Here's how the part is built. I have some questions about the finished solid (model axes, mm). Give positions to 0.01 mm unless a question says otherwise; leave off trailing zeros. Loops run counter-clockwise (first coordinate to the right, second up) from the corner with the lowest first, then second, coordinate; pieces in that order, holes last.
Q1. I need wall thicknesses on probe 1 along Z at (x, y) = (20.5, 3); probe 2 along Z at (x, y) = (0, 4.75); probe 3 along Z at (x, y) = (88, 1). Which ranges of each line are inside material? Lowest first, please.
Q2. I'm going to push flat-ended pins straight in: P1, Ø1, axis at y = 2, z = -40, coming from the +X side; P2, Ø2, axis at y = 3, z = -9, coming from the +X side; P3, Ø3, axis at x = 110, y = 2, coming from the +Z side; P4, Ø4, axis at x = 17.64, z = -49.39, coming from the +Y side. Where does each tip first touch, or does it pass through?
Q3. Suppose I cut it at B-B (z = 0). List the corners of the cut face in (x, y) for me, and give its area (3 significant figures).
Q4. Suppose I cut it at A-A (x = 79.5). List the corners of the cut face in (y, z) for me, and give its area (3 significant figures).
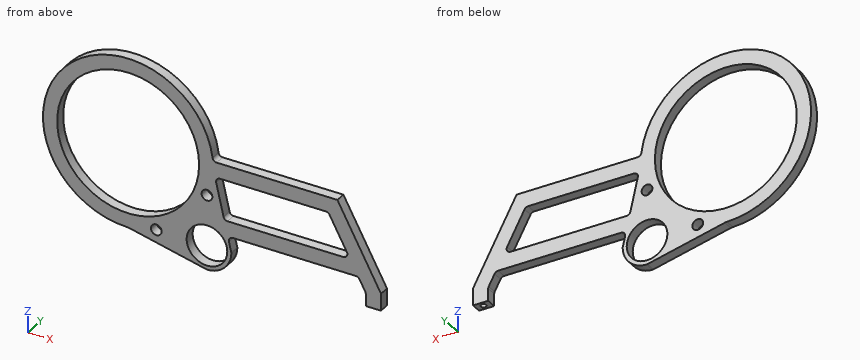
```python
from build123d import *

# Parameters (mm, degrees)
BOSS_EXTRUDE1_DEPTH             = 6.35
FILLET2_R                       = 6.35
BOSS_EXTRUDE2_DEPTH             = 6.35
SKETCH3_R                       = 44.4754
SKETCH3_R_2                     = 12.7254
CUT_EXTRUDE1_DEPTH              = 7.35
FILLET3_R                       = 2.54
F_6_32_TAPPED_HOLE1_D           = 2.7051
F_6_32_TAPPED_HOLE1_DEPTH       = 9.398
F_6_32_TAPPED_HOLE1_CBORE_D     = 3.5052
F_6_32_TAPPED_HOLE1_CBORE_DEPTH = 7.112
F_6_32_TAPPED_HOLE1_TIP         = 0.81269403
F_1_4_CLEARANCE_HOLE1_D         = 6.7564
F_1_4_CLEARANCE_HOLE1_DEPTH     = 25.4
F_1_4_CLEARANCE_HOLE1_TIP       = 2.029827343


with BuildPart() as part:
    # Sketch1 → Boss-Extrude1 (new body)
    with BuildSketch(Plane(origin=(0, 0, 0), x_dir=(1, 0, 0), z_dir=(0, 1, 0))):
        with BuildLine():
            Line((0, 53.3781), (49.391408666, 64.669508666))
            ThreePointArc((49.391408666, 64.669508666), (60.19465678, 60.19465678), (64.669508666, 49.391408666))
            Line((64.669508666, 49.391408666), (53.3781, 0))
            ThreePointArc((53.3781, 0), (-37.744016477, -37.744016477), (0, 53.3781))
        make_face()
    extrude(amount=BOSS_EXTRUDE1_DEPTH)

    # Fillet2
    fillet2_edges = [part.edges().sort_by_distance(p)[0] for p in [
        (0, 3.175, -53.3781),
        (53.3781, 3.175, 0),
    ]]
    fillet(fillet2_edges, radius=FILLET2_R)

    # Sketch4 → Boss-Extrude2 (add)
    with BuildSketch(Plane(origin=(0, 6.35, 0), x_dir=(1, 0, 0), z_dir=(0, 1, 0))):
        Polygon((52.07, -4.84480564), (131.116478857, -4.84480564), (158.4325, 45.95519436), (158.4325, 56.6794421), (148.9075, 56.6794421), (148.9075, 48.353689839), (144.203285679, 39.60519436), (52.07, 39.60519436), (52.07, 30.08019436), (139.081531715, 30.08019436), (125.423521143, 4.68019436), (52.07, 4.68019436), align=None)
    extrude(amount=-BOSS_EXTRUDE2_DEPTH)

    # Sketch3 → Cut-Extrude1 (cut, through all)
    with BuildSketch(Plane(origin=(0, 6.35, 0), x_dir=(1, 0, 0), z_dir=(0, 1, 0))):
        Circle(SKETCH3_R)
        with Locations((49.391408666, 49.391408666)):
            Circle(SKETCH3_R_2)
    extrude(amount=-CUT_EXTRUDE1_DEPTH, mode=Mode.SUBTRACT)

    # Fillet3
    fillet3_edges = [part.edges().sort_by_distance(p)[0] for p in [
        (139.081531715, 3.175, -30.08019436),
        (54.448042903, 3.175, -4.68019436),
        (125.423521143, 3.175, -4.68019436),
        (60.25475682, 3.175, -30.08019436),
        (62.432274539, 3.175, -39.60519436),
        (144.203285679, 3.175, -39.60519436),
        (148.9075, 3.175, -48.353689839),
        (53.157778527, 3.175, 4.84480564),
        (49.391408666, 3.175, -64.669508666),
        (64.669508666, 3.175, -49.391408666),
    ]]
    fillet(fillet3_edges, radius=FILLET3_R)

    # #6-32 Tapped Hole1
    with Locations(Plane(origin=(0, 0, -56.6794421), x_dir=(-1, 0, 0), z_dir=(0, 0, -1))):
        with Locations((-153.67, 3.175)):
            CounterBoreHole(F_6_32_TAPPED_HOLE1_D / 2, F_6_32_TAPPED_HOLE1_CBORE_D / 2, F_6_32_TAPPED_HOLE1_CBORE_DEPTH, depth=F_6_32_TAPPED_HOLE1_DEPTH)
            with Locations((0, 0, -(F_6_32_TAPPED_HOLE1_DEPTH + F_6_32_TAPPED_HOLE1_TIP / 2))):  # 118° drill point
                Cone(0, F_6_32_TAPPED_HOLE1_D / 2, F_6_32_TAPPED_HOLE1_TIP, mode=Mode.SUBTRACT)

    # 1/4 Clearance Hole1
    with Locations(Plane.XZ):
        with Locations((49.391408666, -17.641408666), (17.641408666, -49.391408666)):
            Hole(F_1_4_CLEARANCE_HOLE1_D / 2, depth=F_1_4_CLEARANCE_HOLE1_DEPTH)
            with Locations((0, 0, -(F_1_4_CLEARANCE_HOLE1_DEPTH + F_1_4_CLEARANCE_HOLE1_TIP / 2))):  # 118° drill point
                Cone(0, F_1_4_CLEARANCE_HOLE1_D / 2, F_1_4_CLEARANCE_HOLE1_TIP, mode=Mode.SUBTRACT)


solid = part.part
```
Solutions:
1. probe 1: z = -58.06 to -51.19, -47.59 to -39.47, 39.47 to 49.28
1. probe 2: z = -53.42 to -44.48, 44.48 to 53.38
1. probe 3: z = -39.61 to -30.08, -4.68 to 4.84
2. P1: stops at x = 155.5
2. P2: stops at x = 139.1
2. P3: stops at z = 4.84
2. P4: passes through
3. outline: (-53.38, 0) - (-44.48, 0) - (-44.48, 6.35) - (-53.38, 6.35) - close; (44.48, 0) - (133.72, 0) - (133.72, 6.35) - (44.48, 6.35) - close
3. area: 623 mm2
4. outline: (0, -39.61) - (6.35, -39.61) - (6.35, -30.08) - (0, -30.08) - close; (0, -4.68) - (6.35, -4.68) - (6.35, 4.84) - (0, 4.84) - close
4. area: 121 mm2
